Autodesk Fusion 360 part; units mm, degrees
sketch "Base" plane through (0, 0, 0) normal (0, 0, 1) x (1, 0, 0)
  line L0 (10, -10) -> (-10, -10)
  line L1 (-10, -10) -> (-10, 10)
  line L2 (-10, 10) -> (10, 10)
  line L3 (10, 10) -> (10, -10)
  line L4 (10, -10) -> (-10, 10) construction
  line L5 (-10, -10) -> (10, 10) construction
  circle A0 centre (0, 0) radius 2.25
  dimension "d1" = 20
  dimension "d2" = 20
  dimension "d3" = 4.5
extrude "Extrude1" add sketch "Base" along normal blind 3
extrude "Extrude2" add sketch "Base" along normal blind 10 contours A0
fillet "Fillet1" radius 1.5 4 edges at (10, 0, 0) (0, 10, 0) (-10, 0, 0) (0, -10, 0)
sketch "Inserts" plane through (0, 0, 0) normal (0, 0, 1) x (1, 0, 0)
  line L0 (-10, -10) -> (-3, -10)
  line L1 (-3, -10) -> (3, -10)
  line L2 (3, -10) -> (3, -8)
  line L3 (-3, -10) -> (-3, -8)
  line L4 (-3, -8) -> (-3, -3.6)
  line L5 (-3, -3.6) -> (3, -3.6)
  line L6 (3, -8) -> (5.25, -8)
  line L7 (-3, -8) -> (-5.25, -8)
  line L8 (-5.25, -8) -> (-3, -3.6)
  line L9 (5.25, -8) -> (3, -3.6)
  line L10 (-3, -8) -> (3, -8)
  line L11 (-10, 3) -> (-10, -3)
  line L12 (-8, 3) -> (-3.6, 3)
  line L13 (-8, -3) -> (-8, -5.25)
  line L14 (-3.6, 3) -> (-3.6, -3)
  line L15 (-8, 3) -> (-8, -3)
  line L16 (-8, 5.25) -> (-3.6, 3)
  line L17 (-10, 10) -> (-10, 3)
  line L18 (-8, 3) -> (-8, 5.25)
  line L19 (-8, -5.25) -> (-3.6, -3)
  line L20 (-10, 3) -> (-8, 3)
  line L21 (-10, -3) -> (-8, -3)
  line L22 (3, 10) -> (-3, 10)
  line L23 (3, 8) -> (3, 3.6)
  line L24 (-3, 8) -> (-5.25, 8)
  line L25 (3, 3.6) -> (-3, 3.6)
  line L26 (3, 8) -> (-3, 8)
  line L27 (5.25, 8) -> (3, 3.6)
  line L28 (10, 10) -> (3, 10)
  line L29 (3, 8) -> (5.25, 8)
  line L30 (-5.25, 8) -> (-3, 3.6)
  line L31 (3, 10) -> (3, 8)
  line L32 (-3, 10) -> (-3, 8)
  line L33 (10, -3) -> (10, 3)
  line L34 (8, -3) -> (3.6, -3)
  line L35 (8, 3) -> (8, 5.25)
  line L36 (3.6, -3) -> (3.6, 3)
  line L37 (8, -3) -> (8, 3)
  line L38 (8, -5.25) -> (3.6, -3)
  line L39 (10, -10) -> (10, -3)
  line L40 (8, -3) -> (8, -5.25)
  line L41 (8, 5.25) -> (3.6, 3)
  line L42 (10, -3) -> (8, -3)
  line L43 (10, 3) -> (8, 3)
  point P0 (-10, -10)
  point P1 (-10, 10)
  point P2 (10, 10)
  point P3 (10, -10)
  dimension "d10" = 7
  dimension "d11" = 6
  dimension "d12" = 2
  dimension "d13" = 2
  dimension "d14" = 4.4
  dimension "d15" = 6
  dimension "d16" = 2.25
  dimension "d17" = 2.25
  dimension "d27" = 7
  dimension "d28" = 6
  dimension "d29" = 2
  dimension "d30" = 2
  dimension "d31" = 4.4
  dimension "d32" = 6
  dimension "d33" = 2.25
  dimension "d34" = 2.25
  dimension "d35" = 7
  dimension "d36" = 6
  dimension "d37" = 2
  dimension "d38" = 2
  dimension "d39" = 4.4
  dimension "d40" = 6
  dimension "d41" = 2.25
  dimension "d42" = 2.25
  dimension "d43" = 7
  dimension "d44" = 6
  dimension "d45" = 2
  dimension "d46" = 2
  dimension "d47" = 4.4
  dimension "d48" = 6
  dimension "d49" = 2.25
  dimension "d50" = 2.25
extrude "Extrude4" add sketch "Inserts" along normal blind 3 from surface at 3 contours L4 L7 L8 | L4 L5 L6 L9 L10
extrude "Extrude5" add sketch "Inserts" along normal blind 4.5 from surface at 3 contours L1 L2 L3 L10
extrude "Extrude6" add sketch "Inserts" along normal blind 3 from surface at 3 contours L12 L16 L18 | L12 L13 L14 L15 L19 | L23 L27 L29 | L23 L24 L25 L26 L30 | L34 L38 L40 | L34 L35 L36 L37 L41
extrude "Extrude7" add sketch "Inserts" along normal blind 4.5 from surface at 3 contours L11 L15 L20 L21 | L22 L26 L31 L32 | L33 L37 L42 L43
Here's how the part is built. I have some questions about the finished solid (model axes, mm). A direction names the side the tool comes from. Coordinates: 2 decimals unless noted, no trailing zeros. Write each loop counter-clockwise with the first axis right and the second up, starting at its lowest first coordinate (ties: lowest second). Pieces come first, ordered by that corner, then holes. Notation, with made-up numbers: (69.25, 18.5) - (100.25, 18.5) arc R3 ccw to (100.25, 22.5) - close; hole circle Ø5 at (72, 7.25). An arc over 180 degrees is marked (long way). One line per item, written item: value.
1) Suppose I cut it at B-B on x = 0. Write out the boundary of the cut face in (y, z).
Model answer:
outline: (-10, 1.5) arc R1.5 ccw to (-8.5, 0) - (8.5, 0) arc R1.5 ccw to (10, 1.5) - (10, 7.5) - (8, 7.5) - (8, 6) - (3.6, 6) - (3.6, 3) - (2.25, 3) - (2.25, 10) - (-2.25, 10) - (-2.25, 3) - (-3.6, 3) - (-3.6, 6) - (-8, 6) - (-8, 7.5) - (-10, 7.5) - close
2) Suppose I cut it at A-A on z = 3.25. State how many separate pieces and enclosed holes the cut face has, and give its area (3 significant figures).
Model answer:
separate pieces: 5
enclosed holes: 0
area: 209 mm²
3) We'd pull the mould along Y, two halves only. Please class faces 1 (the flat face through (5.83, 4.14, 4.48)), 2 (the flat face through (9, 3, 5)), 3 (the flat face through (0, 3.6, 4)), 4 (the flat face through (0, 0, 0)): pulls with the +Y half, pulls with the -Y half, needs draft (parallel to the pull), parting line crosses it, or undercut.
Model answer:
face 1: undercut
face 2: pulls with the +Y half
face 3: undercut
face 4: needs draft
4) On a 3-axis mill with a long thin cutter (end or side, diameter ignored), from which of +Z, -Z, +X, -X, +Y, -Y can I reach the whole of each face in a straight line? I mean faces 5 (the flat face through (0, -6, 6)), 6 (the flat face through (4, -8, 4)), 7 (the flat face through (0, -3.6, 4)), 8 (the flat face through (-6, 0, 6)), 9 (the flat face through (3, 9, 5)). Say none if no direction works.
Model answer:
face 5: +Z, +X, -X
face 6: +Z, +X, -Y
face 7: +Z
face 8: +Z, +Y, -Y
face 9: +Z, +X, +Y
5) Suppose I cut it at D-D on z = 7. Write out the boundary of the cut face in (x, y).
Model answer:
outline: (-10, -3) - (-8, -3) - (-8, 3) - (-10, 3) - close; (-3, -10) - (3, -10) - (3, -8) - (-3, -8) - close; (-3, 8) - (3, 8) - (3, 10) - (-3, 10) - close; circle Ø4.5 at (0, 0); (8, -3) - (10, -3) - (10, 3) - (8, 3) - close
6) I'm going to push flat-ended pins straight in: P1, Ø1, axis at y = 8.5, z = 6.5, coming from the -X side; P2, Ø1.8, axis at x = 4.5, z = 4.5, coming from the -Y side; P3, Ø1, axis at x = -6, y = 1, coming from the +Z side. Where does each tip first touch, or does it pass through?
Model answer:
P1: stops at x = -3
P2: stops at y = -8
P3: stops at z = 6
7) I need wall thicknesses on line 1 along X through (y, z) = (2.75, 4.5); line 2 along Z through (x, y) = (-3, -1); line 3 along Z through (x, y) = (2.75, 4.25). Which ranges of each line are inside material? Lowest first, please.
Model answer:
line 1: x = -10 to -3.6, 3.6 to 10
line 2: z = 0 to 3
line 3: z = 0 to 6
